Could you check a few things on this drawing? It's one solid part, dimensions in mm from its lowest x, y, z. Give positions to 0.01 mm unless a question says otherwise; leave off trailing zeros. Order: outer loops, then holes, each group sorted by start corner. A loop starts at its lowest first (then second) coordinate and runs counter-clockwise, first axis right, second up. Notation, with made-up numbers: (59, -28) - (88, -28) arc R23 ccw to (88, -6) - close; hole circle Ø7 at (-10.75, 33.25). An arc over 180 degrees is marked (long way). Answer as CSV lines item,"result".
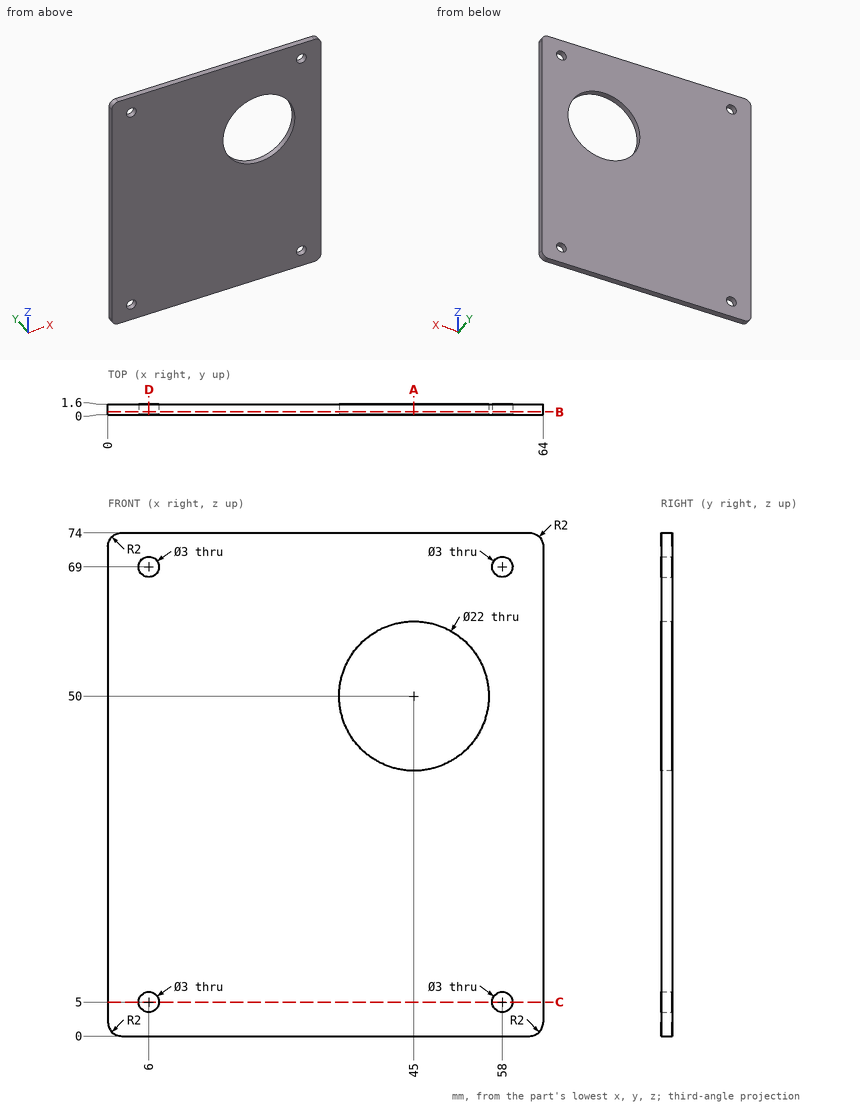
1) I want a section at A-A on x = 45. Write out the boundary of the cut face in (y, z), plus the area to 3 significant figures.
Answer block:
outline,"(0, 0) - (1.6, 0) - (1.6, 39) - (0, 39) - close; (0, 61) - (1.6, 61) - (1.6, 74) - (0, 74) - close"
area,"83.2 mm2"
2) I want a section at B-B on y = 0.45. Write out the boundary of the cut face in (x, z), plus the area to 3 significant figures.
Answer block:
outline,"(0, 2) arc R2 ccw to (2, 0) - (62, 0) arc R2 ccw to (64, 2) - (64, 72) arc R2 ccw to (62, 74) - (2, 74) arc R2 ccw to (0, 72) - close; hole circle Ø3 at (6, 5); hole circle Ø3 at (6, 69); hole circle Ø22 at (45, 50); hole circle Ø3 at (58, 5); hole circle Ø3 at (58, 69)"
area,"4,320 mm2"
3) I want a section at D-D on x = 6. Write out the boundary of the cut face in (y, z).
Answer block:
outline,"(0, 0) - (1.6, 0) - (1.6, 3.5) - (0, 3.5) - close; (0, 6.5) - (1.6, 6.5) - (1.6, 67.5) - (0, 67.5) - close; (0, 70.5) - (1.6, 70.5) - (1.6, 74) - (0, 74) - close"
4) I want a section at C-C on z = 5. Write out the boundary of the cut face in (x, y), plus the area to 3 significant figures.
Answer block:
outline,"(0, 0) - (4.5, 0) - (4.5, 1.6) - (0, 1.6) - close; (7.5, 0) - (56.5, 0) - (56.5, 1.6) - (7.5, 1.6) - close; (59.5, 0) - (64, 0) - (64, 1.6) - (59.5, 1.6) - close"
area,"92.8 mm2"
5) I need wall thicknesses on line 1 along X through (y, z) = (1.1, 5); line 2 along Z through (x, y) = (7, 0.6); line 3 along Z through (x, y) = (5.5, 0.2). Which ranges of each line are inside material? Lowest first, please. Write a range as [from, to].
Answer block:
line 1,"[0, 4.5], [7.5, 56.5], [59.5, 64]"
line 2,"[0, 3.88], [6.12, 67.88], [70.12, 74]"
line 3,"[0, 3.59], [6.41, 67.59], [70.41, 74]"
6) I'm going to push a flat-ended pin straight in: P1, Ø4, axis at x = 58, z = 5, coming from the +Y side. Where does the tip first touch, or does it pass through?
Answer block:
P1,"y = 1.6"
